from build123d import *

# Parameters (mm, degrees)
F0_W        = 173
F0_H        = 120.5
F0_W_2      = 136
F0_H_2      = 114.5
F0_W_3      = 25
F0_H_3      = 110.5
F0_W_4      = 127
F0_H_4      = 101
F1_DEPTH    = 5.9
F3_START    = -0.9
F0_W_5      = 118
F0_H_5      = 92
F1_FACE_W   = 173
F1_FACE_H   = 120.5
F1_FACE_W_2 = 25
F1_FACE_H_2 = 110.5
F1_FACE_W_3 = 127
F1_FACE_H_3 = 101
F3_DEPTH    = 2
F4_START    = 2
F4_DEPTH    = 4


with BuildPart() as f1:
    # F0 (on Front) → F1 (new body)
    with BuildSketch(Plane.XZ):
        with Locations((-17.8190767765, 0)):
            Rectangle(F0_W, F0_H)
        with Locations((-33.3190767765, 0)):
            Rectangle(F0_W_2, F0_H_2, mode=Mode.SUBTRACT)
        with Locations((51.1809232235, 0)):
            Rectangle(F0_W_3, F0_H_3, mode=Mode.SUBTRACT)
        with Locations((-33.3190767765, 0)):
            Rectangle(F0_W_2, F0_H_2)
        with Locations((-31.8190767765, 0)):
            Rectangle(F0_W_4, F0_H_4, mode=Mode.SUBTRACT)
    extrude(amount=F1_DEPTH)

    # F2: F1 across face


with BuildPart() as f1_1:
    add(f1.part)
    add(f1.part.mirror(Plane(origin=(-19.9180876192, 0, 0), x_dir=(1, 0, 0), z_dir=(0, 1, 0))))

    # F0 (on Front) + F1_face (on face) → F3 (join)
    with BuildSketch(Plane.XZ.offset(F3_START)):
        with Locations((-31.8190767765, 0)):
            Rectangle(F0_W_4, F0_H_4)
        with Locations((-31.8190767765, 0)):
            Rectangle(F0_W_5, F0_H_5, mode=Mode.SUBTRACT)
    with BuildSketch(Plane(origin=(-19.9180876192, -5.9, 0), x_dir=(1, 0, 0), z_dir=(0, -1, 0)).offset(F3_START)):
        with Locations((2.0990108427, 0)):
            Rectangle(F1_FACE_W, F1_FACE_H)
        with Locations((71.0990108427, 0)):
            Rectangle(F1_FACE_W_2, F1_FACE_H_2, mode=Mode.SUBTRACT)
        with Locations((-11.9009891573, 0)):
            Rectangle(F1_FACE_W_3, F1_FACE_H_3, mode=Mode.SUBTRACT)
    extrude(amount=-F3_DEPTH)

    # F0 (on Front) → F4 (cut)
    with BuildSketch(Plane.XZ.offset(F4_START)):
        with Locations((-33.3190767765, 0)):
            Rectangle(F0_W_2, F0_H_2)
        with Locations((-31.8190767765, 0)):
            Rectangle(F0_W_4, F0_H_4, mode=Mode.SUBTRACT)
    extrude(amount=F4_DEPTH, mode=Mode.SUBTRACT)


solid = f1_1.part
The model under review builds one solid part; all positions refer to its coordinate system, in mm. A direction names the side the tool comes from. Round coordinates to 2 decimals unless told otherwise and drop trailing zeros. Loops run counter-clockwise (first coordinate to the right, second up) from the corner with the lowest first, then second, coordinate; pieces in that order, holes last. Notation, with made-up numbers: (66.25, 0) -> (92.25, 0) arc R32 cw to (92.25, 34) -> close; hole circle Ø9 at (51, 51). An arc over 180 degrees is marked (long way). Answer as CSV lines item,"result".
1) Draft analysis for pull direction Z (two halves, no side actions). For faces 1 (the face through (-19, 0, -60.25)), 2 (the face through (51, 0, 55.25)), 3 (the face through (-25, -5.9, -58)), 4 (the face through (-37, 0.9, -48)), state which applies: pulls with the +Z half, pulls with the -Z half, needs draft (parallel to the pull), parting line crosses it, or undercut.
Geometry results:
face 1,"pulls with the -Z half"
face 2,"undercut"
face 3,"needs draft"
face 4,"undercut"
2) To check wall thickness, follow line 1 along X through (y, z) = (5.25, 34.5); line 2 along X through (y, z) = (-5, 17); line 3 along Z through (x, y) = (-50, 5.5). State the ranges of each line that lie inside material, in increasing order. Write a range as from..to.
Geometry results:
line 1,"x = -104.32..-95.32, 31.68..38.68, 63.68..68.68"
line 2,"x = -104.32..-101.32, 34.68..38.68, 63.68..68.68"
line 3,"z = -60.25..-50.5, 50.5..60.25"
3) Add section C-C on x = 51. Write out the cut boundary in (y, z), plus the area to 3 significant figures.
Geometry results:
outline,"(-5.9, -60.25) -> (5.9, -60.25) -> (5.9, -55.25) -> (-5.9, -55.25) -> close; (-5.9, 55.25) -> (5.9, 55.25) -> (5.9, 60.25) -> (-5.9, 60.25) -> close"
area,"118 mm²"
4) Add section A-A on x = -27.5. Write out the cut boundary in (y, z).
Geometry results:
outline,"(-5.9, -60.25) -> (5.9, -60.25) -> (5.9, -50.5) -> (2.9, -50.5) -> (2.9, -46) -> (0.9, -46) -> (0.9, -50.5) -> (-2, -50.5) -> (-2, -57.25) -> (-5.9, -57.25) -> close; (-5.9, 57.25) -> (-2, 57.25) -> (-2, 50.5) -> (0.9, 50.5) -> (0.9, 46) -> (2.9, 46) -> (2.9, 50.5) -> (5.9, 50.5) -> (5.9, 60.25) -> (-5.9, 60.25) -> close"
5) Tool access review of faces 5 (the face through (-19, 0, 60.25)), 6 (the face through (68.681, 0, -1)), 7 (the face through (-101.319, -4, -1)), 8 (the face through (-37, 2.9, -48)), 9 (the face through (63.681, 0, -1)): name each direction out of +Z, -Z, +X, -X, +Y, -Y from which nothing blocks a thin tool from reaching the whole face with its end or side.
Geometry results:
face 5,"+Z, +X, -X, +Y, -Y"
face 6,"+Z, -Z, +X, +Y, -Y"
face 7,"-Y"
face 8,"+Y"
face 9,"+Y, -Y"
6) Add section B-B on z = 13.5. Write out the cut boundary in (x, y).
Geometry results:
outline,"(-104.32, -5.9) -> (-101.32, -5.9) -> (-101.32, -2) -> (-95.32, -2) -> (-95.32, 0.9) -> (-90.82, 0.9) -> (-90.82, 2.9) -> (-95.32, 2.9) -> (-95.32, 5.9) -> (-104.32, 5.9) -> close; (27.18, 0.9) -> (31.68, 0.9) -> (31.68, -2) -> (34.68, -2) -> (34.68, -5.9) -> (38.68, -5.9) -> (38.68, 5.9) -> (31.68, 5.9) -> (31.68, 2.9) -> (27.18, 2.9) -> close; (63.68, -5.9) -> (68.68, -5.9) -> (68.68, 5.9) -> (63.68, 5.9) -> close"
7) For P1, Ø12, axis at x = -83.5, z = 26, coming from the -Y side, flat-tipped, find the tip position at first contact; note if it passes through.
Geometry results:
P1,"passes through"
